Design review of the part built by this model. Coordinates are the model's own, in mm. Face numbers are marked on the shaded views. A direction names the side the tool comes from. Round coordinates to 2 decimals unless told otherwise and drop trailing zeros. Write each loop counter-clockwise with the first axis right and the second up, starting at its lowest first coordinate (ties: lowest second). Pieces come first, ordered by that corner, then holes. Notation, with made-up numbers: (-30.5, -20) - (6.5, -20) arc R21 cw to (6.5, -2) - close; hole circle Ø1 at (37, -21.5). An arc over 180 degrees is marked (long way). Use one line per item in the form item = value.
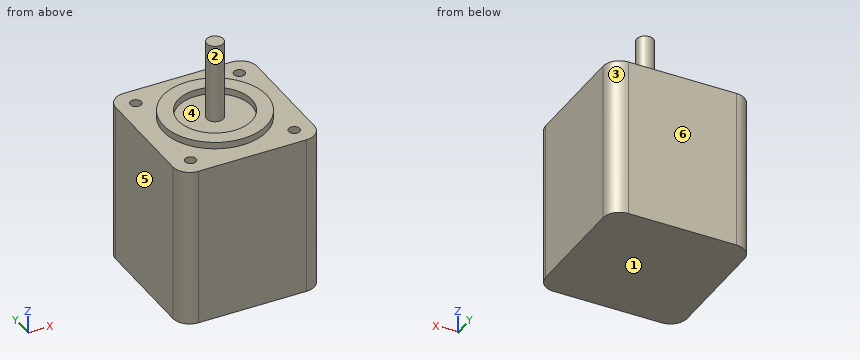
```python
from build123d import *

# Parameters (mm, degrees)
F0_W     = 42.3
F0_H     = 42.3
F1_DEPTH = 48
F2_D     = 3.3
F2_DEPTH = 4.5
F2_TIP   = 0.9914200214
F3_R     = 5
F4_R     = 15.495
F4_R_2   = 11
F5_DEPTH = 2.03
F6_R     = 2.495
F7_DEPTH = 23.88


with BuildPart() as f1:
    # F0 (on Top) → F1 (new body)
    with BuildSketch(Plane.XY):
        Rectangle(F0_W, F0_H)
    extrude(amount=-F1_DEPTH)

    # F2
    with Locations(Plane.XY):
        with Locations((-15.495, 15.495), (-15.495, -15.495), (15.495, -15.495), (15.495, 15.495)):
            Hole(F2_D / 2, depth=F2_DEPTH)
            with Locations((0, 0, -(F2_DEPTH + F2_TIP / 2))):  # 118° drill point
                Cone(0, F2_D / 2, F2_TIP, mode=Mode.SUBTRACT)

    # F3
    f3_edges = [f1.edges().sort_by_distance(p)[0] for p in [
        (-21.15, 21.15, -24),
        (-21.15, -21.15, -24),
        (21.15, -21.15, -24),
        (21.15, 21.15, -24),
    ]]
    fillet(f3_edges, radius=F3_R)

    # F4 (on face) → F5 (join)
    with BuildSketch(Plane.XY):
        Circle(F4_R)
        Circle(F4_R_2, mode=Mode.SUBTRACT)
    extrude(amount=F5_DEPTH)

    # F6 (on face) → F7 (join)
    with BuildSketch(Plane.XY):
        Circle(F6_R)
    extrude(amount=F7_DEPTH)


solid = f1.part
```
Q1. We need section D-D on x = -5. Write out the cut boundary in (y, z).
Calculated:
outline = (-21.15, -48) - (21.15, -48) - (21.15, 0) - (14.67, 0) - (14.67, 2.03) - (9.8, 2.03) - (9.8, 0) - (-9.8, 0) - (-9.8, 2.03) - (-14.67, 2.03) - (-14.67, 0) - (-21.15, 0) - close
Q2. We need section A-A on x = 0. Write out the cut boundary in (y, z) (3 decimals).
Calculated:
outline = (-21.15, -48) - (21.15, -48) - (21.15, 0) - (15.495, 0) - (15.495, 2.03) - (11, 2.03) - (11, 0) - (2.495, 0) - (2.495, 23.88) - (-2.495, 23.88) - (-2.495, 0) - (-11, 0) - (-11, 2.03) - (-15.495, 2.03) - (-15.495, 0) - (-21.15, 0) - close
Q3. For P1, Ø4.5, axis at x = 15.495, y = -15.495, coming from the +Z side; P2, Ø3, axis at x = -15.495, y = -15.495, coming from the +Z side; P3, Ø2, axis at x = -15.495, y = 15.495, coming from the +Z side, all flat-tipped, find the tip position at first contact; note any pin that passes through.
Calculated:
P1 = 0
P2 = -4.59
P3 = -4.89
Q4. To check wall thickness, follow line 1 along Y through (x, z) = (0, 0.45) (3 decimals); line 2 along Z through (x, y) = (11, 10); line 3 along Z through (x, y) = (13, -12). State the ranges of each line that lie inside material, in increasing order. Write a range as from..to.
Calculated:
line_1 = -15.495..-11, -2.495..2.495, 11..15.495
line_2 = -48..2.03
line_3 = -48..0
Q5. Draft analysis for pull direction X (two halves, no side actions). For the marked faces 3, 4, 5 and 6, state which applies: released by +X, released by -X, zero draft, split by the parting line, or undercut.
Calculated:
face_3 = released by +X
face_4 = undercut
face_5 = released by -X
face_6 = zero draft
Q6. We need section B-B on z = -2.5. Write out the cut boundary in (x, y) (3 decimals).
Calculated:
outline = (-21.15, -16.15) arc R5 ccw to (-16.15, -21.15) - (16.15, -21.15) arc R5 ccw to (21.15, -16.15) - (21.15, 16.15) arc R5 ccw to (16.15, 21.15) - (-16.15, 21.15) arc R5 ccw to (-21.15, 16.15) - close; hole circle Ø3.3 at (-15.495, -15.495); hole circle Ø3.3 at (-15.495, 15.495); hole circle Ø3.3 at (15.495, -15.495); hole circle Ø3.3 at (15.495, 15.495)
Q7. Machinability: for the marked faces 1 and 2, which of the approach directions +Z, -Z, +X, -X, +Y, -Y give a long, thin tool a straight path to every point of the face, cutting with its end or side? Answer none if there is none.
Calculated:
face_1 = -Z, +X, -X, +Y, -Y
face_2 = +Z
